from build123d import *

# Parameters (mm, degrees)
PAD011_DEPTH = 4
SKETCH025_R  = 1.5
PAD012_DEPTH = 8
SKETCH026_R  = 0.975
PAD013_DEPTH = 4


with BuildPart() as part:
    # Sketch024 → Pad011 (new body)
    with BuildSketch(Plane.XY):
        with BuildLine():
            ThreePointArc((4.21, 0), (5.71, -1.5), (7.21, 0))
            Line((2.5, 8.850012), (7.21, 0))
            ThreePointArc((2.5, 8.850012), (0, 11.35), (-2.5, 8.850012))
            Line((-7.21, 0), (-2.5, 8.850012))
            ThreePointArc((-7.21, 0), (-5.71, -1.5), (-4.21, 0))
            Line((-4.21, 0), (0, 6))
            Line((0, 6), (4.21, 0))
        make_face()
    extrude(amount=PAD011_DEPTH)

    # Sketch025 (on Face9 of Pad011) → Pad012 (join)
    with BuildSketch(Plane.XY.offset(4)):
        with Locations((0, 8.85)):
            Circle(SKETCH025_R)
    extrude(amount=PAD012_DEPTH)

    # Sketch026 (on Face4 of Pad012) → Pad013 (join)
    with BuildSketch(Plane(origin=(0, 0, 0), x_dir=(1, 0, 0), z_dir=(0, 0, -1))):
        with Locations((-5.71, 0)):
            Circle(SKETCH026_R)
        with Locations((5.71, 0)):
            Circle(SKETCH026_R)
    extrude(amount=PAD013_DEPTH)


with BuildPart() as part_1:
    # Body004 placement: moved
    add(part.part.moved(Location((0, -23.5, 6))))


solid = part_1.part
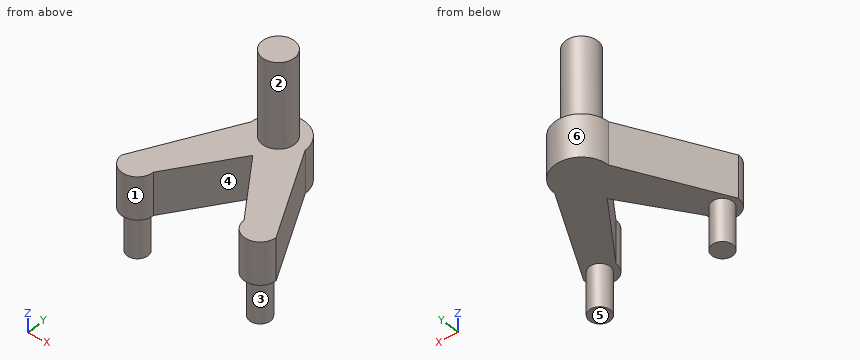
Part model, mm, in its own coordinate system. Face numbers are marked on the shaded views. A direction names the side the tool comes from. Coordinates: 2 decimals unless noted, no trailing zeros. Order: outer loops, then holes, each group sorted by start corner. A loop starts at its lowest first (then second) coordinate and runs counter-clockwise, first axis right, second up.
(1) Tool access for the marked faces 1, 2 and 3: list every direction of +Z, -Z, +X, -X, +Y, -Y with a clear straight run to the whole face (end or side of a thin tool).
Check sheet entries:
face 1: +Z, -Z, -Y
face 2: +Z
face 3: -Z
(2) Slice it at D-D, the plane x = -5.71. Write the cut outline in (y, z) (3 decimals), and give its area (3 significant figures).
Check sheet entries:
outline: (-25, 6) - (-24.475, 6) - (-24.475, 2) - (-22.525, 2) - (-22.525, 6) - (-20.682, 6) - (-20.682, 10) - (-25, 10) - close
area: 25.1 mm2
(3) Pin check, flat tips, straight feed: pin 1 Ø6.5 at (x, y) = (-2.5, -15.5) entering from +Z; pin 2 Ø2 at (x, z) = (1, 10.5) entering from -Y; pin 3 Ø1 at (y, z) = (-23.5, 5) entering from -X (3 decimals); pin 4 Ø8 at (x, z) = (4.5, 16) entering from -Y. Stop position of each tip, or through.
Check sheet entries:
pin 1: stops at z = 18
pin 2: stops at y = -20.16
pin 3: stops at x = -6.685
pin 4: stops at y = -16.06
(4) Pull direction X, two halves, no side cores. Call the marked faces 4, 5 and 6: pulls with the +X half, pulls with the -X half, needs draft (parallel to the pull), parting line crosses it, or undercut.
Check sheet entries:
face 4: undercut
face 5: needs draft
face 6: parting line crosses it
(5) Slice it at A-A, the plane y = -19.25. Write the cut outline in (x, z).
Check sheet entries:
outline: (-4.95, 6) - (-1.23, 6) - (-1.23, 10) - (-4.95, 10) - close; (1.23, 6) - (4.95, 6) - (4.95, 10) - (1.23, 10) - close
(6) Slice it at C-C, the plane x = 6.25. Write the cut outline in (y, z).
Check sheet entries:
outline: (-24.9, 6) - (-24.31, 6) - (-24.31, 2) - (-22.69, 2) - (-22.69, 6) - (-21.7, 6) - (-21.7, 10) - (-24.9, 10) - close
(7) Probe L1, parallel to Z at x = 1.25, y = -18.75; L2, parallel to Y at x = 0, z = 17; L3, parallel to Z at x = 0.75, y = -14. List the from-to ranges inside material, lowest first.
Check sheet entries:
L1: z = 6 to 10
L2: y = -16.15 to -13.15
L3: z = 6 to 18
(8) Slice it at B-B, the plane z = 7. Write the cut outline in (x, y), and give its area (3 significant figures).
Check sheet entries:
outline: (-7.21, -23.5) arc R1.5 ccw to (-4.21, -23.5) - (0, -17.5) - (4.21, -23.5) arc R1.5 ccw to (7.21, -23.5) - (2.5, -14.65) arc R2.5 ccw to (-2.5, -14.65) - close
area: 77.6 mm2
